Input: part model. Units: mm. Frame: model coordinates. A direction names the side the tool comes from. Round coordinates to 2 decimals unless told otherwise and drop trailing zeros. Loops run counter-clockwise (first coordinate to the right, second up) from the corner with the lowest first, then second, coordinate; pieces in that order, holes last. Notation, with made-up numbers: M 43,73 L 47,73 A19 cw 47,106 Z; hole C -18.75,15.5 d7. An arc over 180 degrees is marked long. Use one line per item in the form item = value. Start each with the question number.
Q1. First-contact query: P1, Ø3, axis at x = -2, z = 5.5, coming from the +Y side; P2, Ø1, axis at x = 2, y = -2.5, coming from the +Z side; P3, Ø2, axis at x = -2, z = 10.5, coming from the -Y side. Flat tips, straight axial feed; report the tip coordinate or a pass-through.
Q2. Section query C-C, the plane x = 5.25. Output: boundary loops of the cut face in (y, z) (3 decimals), and give its area (3 significant figures).
Q3. Ray query, line 1 along Y through (x, z) = (0.5, 0) (3 decimals); line 2 along X through (y, z) = (2, -24) (3 decimals); line 3 along Y through (x, z) = (-1.75, 1). Return the intervals inside material, ascending.
Q4. Mould query, pull axis Y, two halves, no side actions, for faces 4 (the flat face through (-3.175, 7, -1)), 5 (the cylindrical face through (-2.392, -24.331, -26.533)), 6 (the cylindrical face through (2.6, 2.8, 1.5)). Classes: pulls with the +Y half, pulls with the -Y half, needs draft (parallel to the pull), parting line crosses it, or undercut.
Q5. Access query for faces 1 (the cylindrical face through (5.52, 9.3, -2.06)), 2 (the cylindrical face through (-0.01, -33.71, -4.43)), 3 (the cylindrical face through (2.37, -24.331, -26.533)). Directions: +Z, -Z, +X, -X, +Y, -Y. A direction counts if a zero-diameter tool reaches every point of the face in a straight line with its end or side. Return the directions, or none.
```python
from build123d import *

# Parameters (mm, degrees)
SKETCH3_R           = 9.525
BOSS_EXTRUDE1_DEPTH = 5
SKETCH4_R           = 3.175
CUT_EXTRUDE1_DEPTH  = 53.161504004
CHAMFER1_SIZE       = 0.25


with BuildPart() as part:
    # Sketch2 → Revolve1 (revolve)
    with BuildSketch(Plane.XY, mode=Mode.PRIVATE) as revolve1_sk:
        Polygon((-3.175, 3.175), (3.175, 3.175), (3.175, 36), (1.5875, 36), (0.833641219, 34), (-0.833641219, 34), (-1.5875, 36), (-3.175, 36), align=None)
    revolve(revolve1_sk.sketch.rotate(Axis((0, 0, 0), (1, 0, 0)), 90), axis=Axis((0, 0, 0), (1, 0, 0)))

    # Sketch3 → Boss-Extrude1 (add)
    with BuildSketch(Plane(origin=(3.175, 0, 0), x_dir=(0, 0, -1), z_dir=(1, 0, 0))):
        with Locations(Location((0, 0, 0), (0, 0, 180))):
            Circle(SKETCH3_R)
    extrude(amount=BOSS_EXTRUDE1_DEPTH)

    # Sketch4 → Cut-Extrude1 (cut, through all)
    with BuildSketch(Plane(origin=(8.175, 0, 0), x_dir=(0, 0, -1), z_dir=(1, 0, 0))):
        with Locations(Location((0, 0, 0), (0, 0, 180))):
            Circle(SKETCH4_R)
    extrude(amount=-CUT_EXTRUDE1_DEPTH, mode=Mode.SUBTRACT)

    # Chamfer1
    chamfer1_edges = [part.edges().sort_by_distance(p)[0] for p in [
        (8.175, 0, -9.525),
        (8.175, 0, -3.175),
        (-3.175, 0, -3.175),
    ]]
    chamfer(chamfer1_edges, length=CHAMFER1_SIZE)


solid = part.part
```
Results found:
q1.P1 = 35.78
q1.P2 = 35.94
q1.P3 = -34.72
q2.outline = C 0,0 d19.05; hole C 0,0 d6.35
q2.area = 253 mm²
q3.line_1 = -34 to -3.175, 3.175 to 34
q3.line_2 = -3.175 to 3.175
q3.line_3 = -35.99 to -3.01, 3.01 to 35.99
q4.face_4 = needs draft
q4.face_5 = parting line crosses it
q4.face_6 = undercut
q5.face_1 = +X
q5.face_2 = none
q5.face_3 = +X, -X
